Solid Edge part; units mm, degrees
sketch "Sketch1" plane through (0, 0, 86.0654) normal (0, 0, 1) x (1, 0, 0)
  line L0 (-64.6, 87.8905) -> (-64.6, 100.0905)
  line L1 (-64.6, 100.0905) -> (-87.5, 100.0905)
  line L2 (-87.5, 100.0905) -> (-87.5, 87.8905)
  line L3 (-87.5, 87.8905) -> (-64.6, 87.8905)
extrude "Protrusion1" add sketch "Sketch1" against normal blind 21
sketch "Sketch2" plane through (-76.05, 93.9905, 86.0654) normal (0, 0, 1) x (1, 0, 0)
  line L0 (2.55, -1.1) -> (2.55, 1.1)
  arc A0 (-2.45, 6.1) -> (2.55, 1.1) centre (-2.45, 1.1) cw
  line L1 (-2.45, 6.1) -> (-6.45, 6.1)
  arc A1 (-11.45, 1.1) -> (-6.45, 6.1) centre (-6.45, 1.1) cw
  line L2 (-11.45, 1.1) -> (-11.45, -1.1)
  arc A2 (-11.45, -1.1) -> (-6.45, -6.1) centre (-6.45, -1.1) ccw
  line L3 (-6.45, -6.1) -> (-2.45, -6.1)
  arc A3 (-2.45, -6.1) -> (2.55, -1.1) centre (-2.45, -1.1) ccw
extrude "ExtrudedProtrusion_5" add sketch "Sketch2" along normal blind 7.5
sketch "Sketch3" plane through (-80.5, 93.9905, 93.5654) normal (0, 0, 1) x (1, 0, 0)
  circle A0 centre (-0.95, 0) radius 2.5
extrude "ExtrudedProtrusion_6" add sketch "Sketch3" along normal blind 4
sketch "Sketch4" plane through (-76.05, 93.9905, 83.3654) normal (0, 0, -1) x (1, 0, 0)
  line L0 (-16.7, -6.1) -> (-11.45, -6.1)
  line L1 (-11.45, -6.1) -> (-11.45, 6.1)
  line L2 (-11.45, 6.1) -> (-16.7, 6.1)
  line L3 (-16.7, 6.1) -> (-16.7, -6.1)
  circle A0 centre (-14, 0) radius 1.1
  line L4 (11.45, -6.1) -> (11.45, 6.1)
  line L5 (11.45, 6.1) -> (16.7, 6.1)
  line L6 (16.7, 6.1) -> (16.7, -6.1)
  line L7 (16.7, -6.1) -> (11.45, -6.1)
  circle A1 centre (14, 0) radius 1.1
extrude "ExtrudedProtrusion_7" add sketch "Sketch4" against normal blind 2.7
Check sheet for the modelled part. Datum: model origin and axes. Units: mm. A direction names the side the tool comes from. Give positions to 0.01 mm unless a question says otherwise; leave off trailing zeros. Loops run counter-clockwise (first coordinate to the right, second up) from the corner with the lowest first, then second, coordinate; pieces in that order, holes last. Notation, with made-up numbers: M -21,-39.75 L -8,-39.75 A28 cw -8,-18.75 Z; hole C 61.5,35.5 d9. An arc over 180 degrees is marked long. Answer as a JSON object with one key per item and string values. Group by question number.
Q1. Release check for a two-part mould opening along X. For faces 1 (the cylindrical face through (-74.93, 89.39, 89.76)), 2 (the cylindrical face through (-62.288, 95.064, 84.696)), 3 (the flat face through (-92.75, 94, 85)), 4 (the cylindrical face through (-90.923, 94.66, 84.696)) record: released by +X, released by -X, zero draft, split by the parting line, or undercut.
Q2. Cross-section at C-C on x = -81.45. Record the cut outline in (y, z).
Q3. Material ranges on line 1 along Y through (x, z) = (-90.05, 85.2); line 2 along X through (y, z) = (93.75, 84.5); line 3 along X through (y, z) = (95.5, 68.5), recorded low to high. Write a range as [from, to].
Q4. Cross-section at A-A on x = -62.05. Record the cut outline in (y, z).
Q5. Cross-section at B-B on z = 91. Record the cut outline in (x, y).
Q6. Go/stop test with flat-tipped pins: P1, Ø4, axis at x = -62.5, y = 96.5, coming from the -Z side; P2, Ø1.5, axis at y = 92, z = 70.5, coming from the -X side; P3, Ø6, axis at y = 94, z = 75, coming from the +X side; P4, Ø6, axis at x = -88.5, z = 87, coming from the -Y side. Record where each tip stops, or that it passes through.
Q7. Access from +Z, -Z, +X, -X, +Y, -Y to the whole of each face (thin tool, end or side, straight path). Record for faces 5 (the flat face through (-64.6, 94, 74)), 6 (the flat face through (-91.3, 94.1, 83.365)), 7 (the flat face through (-79, 92.7, 93.565)), 8 (the cylindrical face through (-86.07, 98.59, 89.76)).
Q8. Cross-section at D-D on y = 98.25. Record the cut outline in (x, z).
Evaluation:
{
 "1": {"face 1": "released by +X", "face 2": "undercut", "face 3": "released by -X", "face 4": "undercut"},
 "2": {"outline": "M 87.89,65.07 L 100.09,65.07 L 100.09,93.57 L 96.49,93.57 L 96.49,97.57 L 91.49,97.57 L 91.49,93.57 L 87.89,93.57 Z"},
 "3": {"line 1": "y = [87.89, 92.89], [95.09, 100.09]", "line 2": "x = [-92.75, -91.12], [-88.98, -63.12], [-60.98, -59.35]", "line 3": "x = [-87.5, -64.6]"},
 "4": {"outline": "M 87.89,83.37 L 92.89,83.37 L 92.89,86.07 L 87.89,86.07 Z; M 95.09,83.37 L 100.09,83.37 L 100.09,86.07 L 95.09,86.07 Z"},
 "5": {"outline": "M -87.5,92.89 A5 ccw -82.5,87.89 L -78.5,87.89 A5 ccw -73.5,92.89 L -73.5,95.09 A5 ccw -78.5,100.09 L -82.5,100.09 A5 ccw -87.5,95.09 Z"},
 "6": {"P1": "stops at z = 83.37", "P2": "stops at x = -87.5", "P3": "stops at x = -64.6", "P4": "stops at y = 87.89"},
 "7": {"face 5": "-Z, +X, +Y, -Y", "face 6": "-Z, -X, +Y, -Y", "face 7": "+Z", "face 8": "+Z, -X, +Y"},
 "8": {"outline": "M -92.75,83.37 L -87.5,83.37 L -87.5,65.07 L -64.6,65.07 L -64.6,83.37 L -59.35,83.37 L -59.35,86.07 L -74.62,86.07 L -74.62,93.57 L -86.38,93.57 L -86.38,86.07 L -92.75,86.07 Z"}
}
